Can you work these out from the model? Positions are in its coordinate system, mm. A direction names the side the tool comes from. Give positions to 0.01 mm unless a question says otherwise; leave off trailing zeros. Write each loop counter-clockwise with the first axis right and the second up, starting at its lowest first coordinate (ties: lowest second). Pieces come first, ordered by that corner, then holes.
```python
from build123d import *

# Parameters (mm, degrees)
F0_R      = 2
F1_DEPTH  = 10
F2_R      = 5
F4_R      = 2
F5_DEPTH  = 10
F7_R      = 5
F7_2_R    = 5
F8_R      = 2
F8_2_R    = 2
F10_DEPTH = 25
F11_R     = 1.5
F12_R     = 1.75
F13_DEPTH = 12.5
F15_W     = 9
F15_H     = 20
F16_DEPTH = 10
F17_W     = 6
F17_H     = 20
F18_DEPTH = 25
F21_R     = 2
F22_DEPTH = 30
F24_R     = 2
F25_DEPTH = 12.5
F27_R     = 2
F28_R     = 2
F29_DEPTH = 8
F30_R     = 2
F31_R     = 2
F32_R     = 1.75
F33_DEPTH = 25
F32_R_2   = 2
F37_ANGLE = 90
F40_W     = 60
F40_H     = 10
F40_R     = 2
F41_DEPTH = 8
F43_R     = 1.5


with BuildPart() as f1:
    # F0 (on Top) → F1 (new body)
    with BuildSketch(Plane.XY):
        Polygon((0, 70), (0, 75), (-20, 75), (-30, 75), (-50, -75), (-40, -75), (0, -75), (0, -65), (-38.6666666667, -65), (-30.8, -6), (0, -6), (0, 0), (0, 6), (-29.2, 6), (-21.3333333333, 65), (0, 65), align=None)
        with Locations((-15, 0)):
            Circle(F0_R, mode=Mode.SUBTRACT)
        with Locations((-10.4101235047, 70)):
            Circle(F0_R, mode=Mode.SUBTRACT)
    extrude(amount=F1_DEPTH)

    # F2
    f2_edges = [f1.edges().sort_by_distance(p)[0] for p in [
        (-21.333333, 65, 5),
        (-30.8, -6, 5),
        (-29.2, 6, 5),
        (-38.666667, -65, 5),
        (-50, -75, 5),
    ]]
    fillet(f2_edges, radius=F2_R)

    # F3: F1 across plane


with BuildPart() as f1_1:
    add(f1.part)
    add(f1.part.mirror(Plane.YZ))

    # F4 (on Top) → F5 (join)
    with BuildSketch(Plane.XY):
        with BuildLine():
            Line((0, 80), (0, 75))
            Line((0, 75), (10, 75))
            Line((10, 75), (30, 75))
            Line((30, 75), (13.3333333333, 200))
            Line((13.3333333333, 200), (4.5, 200))
            Line((4.5, 200), (4.5, 192))
            ThreePointArc((4.5, 192), (3.1819805153, 188.8180194847), (0, 187.5))
            Line((0, 187.5), (0, 170.1721444783))
            Line((0, 170.1721444783), (7.3103807362, 170.1721444783))
            Line((7.3103807362, 170.1721444783), (10, 150))
            Line((10, 150), (18.6666666667, 85))
            Line((18.6666666667, 85), (10, 85))
            Line((10, 85), (0, 85))
            Line((0, 85), (0, 80))
        make_face()
        with Locations((10, 80)):
            Circle(F4_R, mode=Mode.SUBTRACT)
    extrude(amount=F5_DEPTH)


with BuildPart() as f6_1:
    # F6: instance of F1
    add(f1_1.part.mirror(Plane.YZ))

    # F7
    f7_edges = [f6_1.edges().sort_by_distance(p)[0] for p in [
        (-7.310381, 170.172144, 5),
        (-18.666667, 85, 5),
        (-13.333333, 200, 5),
    ]]
    fillet(f7_edges, radius=F7_R)

    # F8#2
    f8_2_edges = [f6_1.edges().sort_by_distance(p)[0] for p in [
        (-4.5, 200, 5),
    ]]
    fillet(f8_2_edges, radius=F8_2_R)


with BuildPart() as f1_2:
    add(f1_1.part)

    # F7#2
    f7_2_edges = [f1_2.edges().sort_by_distance(p)[0] for p in [
        (7.310381, 170.172144, 5),
        (18.666667, 85, 5),
        (13.333333, 200, 5),
    ]]
    fillet(f7_2_edges, radius=F7_2_R)

    # F8
    f8_edges = [f1_2.edges().sort_by_distance(p)[0] for p in [
        (4.5, 200, 5),
    ]]
    fillet(f8_edges, radius=F8_R)

    add(f6_1.part)  # F10 merges F6_1
    # F9 (on Top) → F10 (join)
    with BuildSketch(Plane.XY):
        Polygon((0, -6), (0, 0), (0, 6), (-6, 6), (-6, -6), align=None)
    extrude(amount=F10_DEPTH)

    # F11
    f11_edges = [f1_2.edges().sort_by_distance(p)[0] for p in [
        (-6, -6, 17.5),
        (-6, 0, 25),
        (-3, -6, 25),
        (-6, 6, 17.5),
        (-3, 6, 25),
    ]]
    fillet(f11_edges, radius=F11_R)


with BuildPart() as f13:
    # F12 (on Right) → F13 (new body, symmetric)
    with BuildSketch(Plane.YZ):
        with Locations((0, 20)):
            Circle(F12_R)
    extrude(amount=F13_DEPTH, both=True)


with BuildPart() as f13b:
    # F12 (on Right) → F13, piece 2 (new body, symmetric)
    with BuildSketch(Plane.YZ):
        with Locations((0, 15)):
            Circle(F12_R)
    extrude(amount=F13_DEPTH, both=True)


with BuildPart() as f1_3:
    add(f1_2.part)

    # F14: cut F13b, F13
    add(f13b.part, mode=Mode.SUBTRACT)
    add(f13.part, mode=Mode.SUBTRACT)


with BuildPart() as f16:
    # F15 (on Top) → F16 (new body)
    with BuildSketch(Plane.XY):
        Polygon((0, 65), (15, 65), (15, 85), (0, 85), (0, 75), align=None)
        Polygon((-6, 65), (0, 65), (0, 75), (0, 85), (-6, 85), align=None)
        with Locations((-10.5, 75)):
            Rectangle(F15_W, F15_H)
    extrude(amount=F16_DEPTH)


with BuildPart() as f18:
    # F17 (on Top) → F18 (new body)
    with BuildSketch(Plane.XY):
        with Locations((-3, 75)):
            Rectangle(F17_W, F17_H)
    extrude(amount=F18_DEPTH)


with BuildPart() as f16_1:
    add(f16.part)

    # F19: union F18
    add(f18.part)


with BuildPart() as f16_2:
    # F20: moved
    add(f16_1.part.moved(Location((0, 0, 10))))


with BuildPart() as f22:
    # F21 (on Top) → F22 (new body)
    with BuildSketch(Plane.XY):
        with Locations((-10, 80)):
            Circle(F21_R)
    extrude(amount=F22_DEPTH)


with BuildPart() as f22b:
    # F21 (on Top) → F22, piece 2 (new body)
    with BuildSketch(Plane.XY):
        with Locations((10, 80)):
            Circle(F21_R)
    extrude(amount=F22_DEPTH)


with BuildPart() as f22c:
    # F21 (on Top) → F22, piece 3 (new body)
    with BuildSketch(Plane.XY):
        with Locations((-10.4, 70)):
            Circle(F21_R)
    extrude(amount=F22_DEPTH)


with BuildPart() as f22d:
    # F21 (on Top) → F22, piece 4 (new body)
    with BuildSketch(Plane.XY):
        with Locations((10.4, 70)):
            Circle(F21_R)
    extrude(amount=F22_DEPTH)


with BuildPart() as f16_3:
    add(f16_2.part)

    # F23: cut F22d, F22c, F22b, F22
    add(f22d.part, mode=Mode.SUBTRACT)
    add(f22c.part, mode=Mode.SUBTRACT)
    add(f22b.part, mode=Mode.SUBTRACT)
    add(f22.part, mode=Mode.SUBTRACT)


with BuildPart() as f25:
    # F24 (on Right) → F25 (new body, symmetric)
    with BuildSketch(Plane.YZ):
        with Locations((80, 27.2266920656)):
            Circle(F24_R)
    extrude(amount=F25_DEPTH, both=True)


with BuildPart() as f25b:
    # F24 (on Right) → F25, piece 2 (new body, symmetric)
    with BuildSketch(Plane.YZ):
        with Locations((70, 27.2266920656)):
            Circle(F24_R)
    extrude(amount=F25_DEPTH, both=True)


with BuildPart() as f16_4:
    add(f16_3.part)

    # F26: cut F25b, F25
    add(f25b.part, mode=Mode.SUBTRACT)
    add(f25.part, mode=Mode.SUBTRACT)

    # F27
    f27_edges = [f16_4.edges().sort_by_distance(p)[0] for p in [
        (-6, 65, 27.5),
        (-3, 65, 35),
        (-10.5, 65, 20),
        (-15, 65, 15),
        (7.5, 65, 20),
        (15, 65, 15),
        (15, 75, 10),
        (-15, 75, 10),
        (-6, 75, 35),
        (-10.5, 85, 20),
        (-15, 85, 15),
        (-6, 85, 27.5),
        (-3, 85, 35),
        (7.5, 85, 20),
        (15, 85, 15),
    ]]
    fillet(f27_edges, radius=F27_R)


with BuildPart() as f29:
    # F28 (on Right) → F29 (new body)
    with BuildSketch(Plane.YZ):
        Polygon((-6, 10), (0, 10), (6, 10), (6, 25), (65, 35), (65, 20), (75, 20), (85, 20), (85, 35), (85, 120), (75, 120), (-6, 25), align=None)
        Polygon((17.4430621123, 37.0821219176), (23.9249371816, 44.6843210729), (75, 104.5871725266), (75, 45), (64.1585427985, 45), (51.9163602293, 42.9250538018), align=None, mode=Mode.SUBTRACT)
        with Locations((80, 95)):
            Circle(F28_R, mode=Mode.SUBTRACT)
        with Locations((80, 110)):
            Circle(F28_R, mode=Mode.SUBTRACT)
    extrude(amount=F29_DEPTH)

    # F30
    f30_edges = [f29.edges().sort_by_distance(p)[0] for p in [
        (4, 75, 104.587173),
        (4, 75, 45),
        (4, 17.443062, 37.082122),
        (4, 65, 35),
        (4, 6, 25),
        (4, -6, 25),
    ]]
    fillet(f30_edges, radius=F30_R)

    # F31
    f31_edges = [f29.edges().sort_by_distance(p)[0] for p in [
        (8, 46.246648, 70.864105),
        (8, 34.73905, 72.780367),
        (8, 35.165784, 29.943353),
        (8, 85, 70),
    ]]
    fillet(f31_edges, radius=F31_R)


with BuildPart() as f33:
    # F32 (on Right) → F33 (new body)
    with BuildSketch(Plane.YZ):
        with Locations((0, 20)):
            Circle(F32_R)
    extrude(amount=F33_DEPTH)


with BuildPart() as f33b:
    # F32 (on Right) → F33, piece 2 (new body)
    with BuildSketch(Plane.YZ):
        with Locations((0, 15)):
            Circle(F32_R)
    extrude(amount=F33_DEPTH)


with BuildPart() as f33c:
    # F32 (on Right) → F33, piece 3 (new body)
    with BuildSketch(Plane.YZ):
        with Locations((70, 27.25)):
            Circle(F32_R_2)
    extrude(amount=F33_DEPTH)


with BuildPart() as f33d:
    # F32 (on Right) → F33, piece 4 (new body)
    with BuildSketch(Plane.YZ):
        with Locations((80, 27.25)):
            Circle(F32_R_2)
    extrude(amount=F33_DEPTH)


with BuildPart() as f29_1:
    add(f29.part)

    # F34: cut F33d, F33c, F33b, F33
    add(f33d.part, mode=Mode.SUBTRACT)
    add(f33c.part, mode=Mode.SUBTRACT)
    add(f33b.part, mode=Mode.SUBTRACT)
    add(f33.part, mode=Mode.SUBTRACT)


with BuildPart() as f29_2:
    # F37: moved
    add(f29_1.part.rotate(Axis((0, -39.3833108246, 0), (0, -1, 0)), F37_ANGLE))


with BuildPart() as f29_3:
    # F38: moved
    add(f29_2.part.moved(Location((120, -60, 0))))


with BuildPart() as f39_1:
    # F39: instance of F29
    add(f29_3.part.mirror(Plane.YZ))


with BuildPart() as f41:
    # F40 (on Top) → F41 (new body)
    with BuildSketch(Plane.XY):
        with Locations((0, 20)):
            Rectangle(F40_W, F40_H)
        with Locations((-25, 20)):
            Circle(F40_R, mode=Mode.SUBTRACT)
        with Locations((-10, 20)):
            Circle(F40_R, mode=Mode.SUBTRACT)
        with Locations((10, 20)):
            Circle(F40_R, mode=Mode.SUBTRACT)
        with Locations((25, 20)):
            Circle(F40_R, mode=Mode.SUBTRACT)
    extrude(amount=F41_DEPTH)


with BuildPart() as f41_1:
    # F42: moved
    add(f41.part.moved(Location((0, 0, 8))))

    # F43
    f43_edges = [f41_1.edges().sort_by_distance(p)[0] for p in [
        (0, 15, 8),
        (30, 15, 12),
        (30, 25, 12),
        (30, 20, 8),
        (-30, 20, 8),
        (-30, 15, 12),
        (-30, 25, 12),
        (0, 25, 8),
    ]]
    fillet(f43_edges, radius=F43_R)


with BuildPart() as f29_4:
    # F45: moved
    add(f29_3.part.moved(Location((-50, 0, 0))))


solid = f29_4.part
```
1) For faces 4 (the face through (60, -60, 4)), 5 (the face through (40.122, -25.219, 2.958)), 6 (the face through (25, 9, 3)), which set-ups out of +Z, -Z, +X, -X, +Y, -Y let a thin tool reach every point of the face, with its end or its side?
Values follow:
face 4: +Z, -Z, +X, +Y, -Y
face 5: +Z, -Z, +X
face 6: +Z, -Z
2) Suppose I cut it at B-B on y = 20. Write out the boundary of the cut face in (x, z), plus the area to 3 significant figures.
Values follow:
outline: (-50, 0) - (-42, 0) - (-42, 8) - (-50, 8) - close; (-38, 0) - (-27, 0) - (-27, 8) - (-38, 8) - close; (-23, 0) - (40.75, 0) - (40.75, 8) - (-23, 8) - close; (44.75, 0) - (50, 0) - (50, 8) - (44.75, 8) - close
area: 704 mm2
3) For pin 1 Ø3 at (x, y) = (50, -60) entering from +Z; pin 2 Ø3 at (y, z) = (11.5, 2.5) entering from -X; pin 3 Ø4 at (y, z) = (-7, 3) entering from -X; pin 4 Ø4 at (y, z) = (15.5, 2) entering from +X, each with a flat end and sliding along its axis, tell me the tip position at first contact or that it passes through.
Values follow:
pin 1: passes through
pin 2: stops at x = -47.65
pin 3: stops at x = -26.54
pin 4: stops at x = 50
4) Suppose I cut it at C-C on z = 4.75. Write out the boundary of the cut face in (x, y), plus the area to 3 significant figures.
Values follow:
outline: (-50, 15) - (44.44, -65.52) arc R2 ccw to (45.74, -66) - (60, -66) - (60, -54) - (46.69, -54) arc R2 cw to (44.72, -52.33) - (35.4, 2.67) arc R2 cw to (37.37, 5) - (50, 5) - (50, 25) - (-50, 25) - close; hole circle Ø4 at (-40, 20); hole (-30.46, 11.48) - (28.73, -38.98) arc R2 ccw to (32, -37.13) - (25, 4.16) - (25, 13) arc R2 ccw to (23, 15) - (-29.16, 15) arc R2 ccw to start; hole circle Ø4 at (-25, 20); hole circle Ø4 at (42.75, 10); hole circle Ø4 at (42.75, 20); hole circle Ø3.5 at (50, -60); hole circle Ø3.5 at (55, -60)
area: 3,060 mm2
5) Suppose I cut it at A-A on x = 55. Write out the boundary of the cut face in (y, z), plus the area to 3 significant figures.
Values follow:
outline: (-66, 0) - (-61.75, 0) - (-61.75, 8) - (-64, 8) arc R2 ccw to (-66, 6) - close; (-58.25, 0) - (-54, 0) - (-54, 6) arc R2 ccw to (-56, 8) - (-58.25, 8) - close
area: 66.3 mm2
6) Suppose I cut it at D-D on x = -25. State how many separate pieces and enclosed holes the cut face has, plus the area to 3 significant figures.
Values follow:
separate pieces: 3
enclosed holes: 0
area: 149 mm2
7) Please list where these lines run through material, in increasing order: L1, parallel to X at y = 20, z = 2.25; L2, parallel to X at y = -60, z = 4.25; L3, parallel to X at y = 10, z = 5.5.
Values follow:
L1: x = -50 to -42, -38 to -27, -23 to 40.75, 44.75 to 50
L2: x = 37.96 to 48.25, 51.75 to 53.25, 56.75 to 60
L3: x = -44.14 to -28.72, 25 to 40.75, 44.75 to 50
8) If we mould it in two halves opening along X, with no side actions, what happens to faces 1 (the face through (39.4, -24.55, 7.43)), 2 (the face through (-23, 20, 4)), 3 (the face through (44, 5, 3))? For each: +X half, -X half, draft (parallel to the pull), parting line (faces both ways), or undercut.
Values follow:
face 1: +X half
face 2: undercut
face 3: draft
